Source: CAD feature listing. Evaluate the final solid. Frame: model axes, mm. Round coordinates to 2 decimals unless told otherwise and drop trailing zeros. Write each loop counter-clockwise with the first axis right and the second up, starting at its lowest first coordinate (ties: lowest second). Pieces come first, ordered by that corner, then holes. Notation, with made-up numbers: M 25.25,-4 L 77.25,-4 A15 cw 77.25,20 Z; hole C 86,15 d9. An arc over 180 degrees is marked long. Answer in a Markdown table with one row per item.
from build123d import *

# Parameters (mm, degrees)
F0_W     = 93.98
F0_H     = 93.98
F1_DEPTH = 2.54
F3_DEPTH = 3.81
F4_R     = 5.08


with BuildPart() as f1:
    # F0 (on Top) → F1 (new body)
    with BuildSketch(Plane.XY):
        Rectangle(F0_W, F0_H)
    extrude(amount=F1_DEPTH)

    # F2 (on Top) → F3 (join)
    with BuildSketch(Plane.XY):
        Polygon((-44.45, -44.45), (0, -44.45), (44.45, -44.45), (44.45, 44.45), (-44.45, 44.45), align=None)
    extrude(amount=-F3_DEPTH)

    # F4
    f4_edges = [f1.edges().sort_by_distance(p)[0] for p in [
        (44.45, -44.45, -1.905),
        (-44.45, -44.45, -1.905),
        (-44.45, 44.45, -1.905),
        (44.45, 44.45, -1.905),
        (-46.99, -46.99, 1.27),
        (46.99, -46.99, 1.27),
        (46.99, 46.99, 1.27),
        (-46.99, 46.99, 1.27),
    ]]
    fillet(f4_edges, radius=F4_R)


solid = f1.part
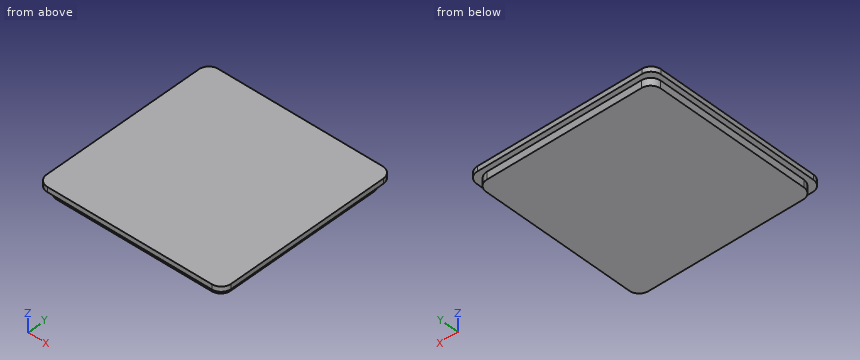
Q1. Contact query for flat-ended pins moving along their axis: pin 1 Ø1.5 at (x, z) = (26, -3) entering from +Y; pin 2 Ø1.9 at (x, z) = (-2.5, -2.5) entering from -Y. Output: stop coordinate, or through.
Solutions:
| item | result |
|---|---|
| pin 1 | stops at y = 44.45 |
| pin 2 | stops at y = -44.45 |
Q2. Material intervals for probe 1 along Y at (x, z) = (21.5, -0.25); probe 2 along Y at (x, z) = (42.5, -0.5), sorted ascending.
Solutions:
| item | result |
|---|---|
| probe 1 | y = -44.45 to 44.45 |
| probe 2 | y = -43.37 to 43.37 |
Q3. Section B-B (y = 11.5). Return loops of the section in (x, z), and give its area (3 significant figures).
Solutions:
| item | result |
|---|---|
| outline | M -46.99,0 L -44.45,0 L -44.45,-3.81 L 44.45,-3.81 L 44.45,0 L 46.99,0 L 46.99,2.54 L -46.99,2.54 Z |
| area | 577 mm2 |
Q4. Section A-A (z = -1.5). Return loops of the section in (x, y), and give its area (3 significant figures).
Solutions:
| item | result |
|---|---|
| outline | M -44.45,-39.37 A5.08 ccw -39.37,-44.45 L 39.37,-44.45 A5.08 ccw 44.45,-39.37 L 44.45,39.37 A5.08 ccw 39.37,44.45 L -39.37,44.45 A5.08 ccw -44.45,39.37 Z |
| area | 7,880 mm2 |
